The model under review builds one solid part; all positions refer to its coordinate system, in mm. Round coordinates to 2 decimals unless told otherwise and drop trailing zeros. Write each loop counter-clockwise with the first axis right and the second up, starting at its lowest first coordinate (ties: lowest second). Pieces come first, ordered by that corner, then holes. Notation, with made-up numbers: M 39.5,-13 L 61.5,-13 A28 cw 61.5,8 Z; hole C -8.75,7.25 d3. An arc over 180 degrees is marked long. Write item = value, one per line. Start each with the question number.
Item 1: Take a section at A-A, the plane x = 43.5. Give the boundary of the cut face in (y, z), plus the area to 3 significant figures.
Item 2: To check wall thickness, follow line 1 along X through (y, z) = (32, 78); line 2 along X through (y, z) = (31.45, 78); line 3 along X through (y, z) = (31.8, 93). State the ranges of each line that lie inside material, in increasing order.
Item 3: Take a section at C-C, the plane x = 68.5. Give the boundary of the cut face in (y, z).
Item 4: For pin 1 Ø2 at (x, z) = (43.5, 3.5) entering from -Y, flat-tipped, find the tip position at first contact; note if it passes through.
Item 5: Take a section at D-D, the plane y = 31.05. Give the boundary of the cut face in (x, z).
Item 6: Take a section at B-B, the plane z = 102.5. Give the boundary of the cut face in (x, y).
from build123d import *
from build123d.topology import SkipClean

# Parameters (mm, degrees)
SKETCH1_R                      = 40
SKETCH1_R_2                    = 38
BOSS_EXTRUDE1_DEPTH            = 200
SKETCH2_R                      = 40
BOSS_EXTRUDE2_DEPTH            = 2
BOSS_EXTRUDE3_DEPTH            = 107
BOSS_EXTRUDE4_DEPTH            = 2
SKETCH5_R                      = 1.75
CUT_EXTRUDE1_DEPTH             = 226.077764339
CUT_EXTRUDE2_REACH             = 218.296
SKETCH6_R                      = 4
CUT_EXTRUDE2_DIRECTION_2_REACH = 218.296
CIRPATTERN1_COUNT              = 2
CIRPATTERN1_ANGLE              = 90
BOSS_EXTRUDE5_REACH            = 241.742
BOSS_EXTRUDE5_END_RADIUS       = 40
SKETCH7_W                      = 14
SKETCH7_H                      = 2
CUT_EXTRUDE3_REACH             = 221.073
SKETCH8_R                      = 1.75
FILLET1_R                      = 3
CUT_EXTRUDE4_REACH             = 220.598
SKETCH9_R                      = 0.25
BOSS_EXTRUDE6_START            = 2
BOSS_EXTRUDE6_DEPTH            = 2
SKETCH11_R                     = 38
CUT_EXTRUDE5_DEPTH             = 219.146739623
CUT_EXTRUDE6_DEPTH             = 2


with BuildPart() as part:
    # Sketch1 → Boss-Extrude1 (new body)
    with BuildSketch(Plane.XY):
        Circle(SKETCH1_R)
        Circle(SKETCH1_R_2, mode=Mode.SUBTRACT)
    extrude(amount=BOSS_EXTRUDE1_DEPTH)

    # Sketch2 → Boss-Extrude2 (add)
    with BuildSketch(Plane.XY.offset(180)):
        Circle(SKETCH2_R)
    extrude(amount=BOSS_EXTRUDE2_DEPTH)

    # Sketch3 → Boss-Extrude3 (add)
    with BuildSketch(Plane(origin=(0, 0, 0), x_dir=(-1, 0, 0), z_dir=(0, 0, -1))):
        with BuildLine():
            Line((-21.071307506, -34), (-72, -34))
            Line((-72, -34), (-72, -30))
            Line((-72, -30), (-26.457513111, -30))
            ThreePointArc((-26.457513111, -30), (-23.848421275, -32.113125085), (-21.071307506, -34))
        make_face()
        with BuildLine():
            Line((-21.071307506, 34), (-72, 34))
            Line((-72, 34), (-72, 30))
            Line((-72, 30), (-26.457513111, 30))
            ThreePointArc((-26.457513111, 30), (-23.848421275, 32.113125085), (-21.071307506, 34))
        make_face()
    extrude(amount=-BOSS_EXTRUDE3_DEPTH)

    # Sketch4 → Boss-Extrude4 (add)
    with BuildSketch(Plane.XY.offset(107)):
        with BuildLine():
            Line((72, -34), (21.071307506, -34))
            ThreePointArc((21.071307506, -34), (40, 0), (21.071307506, 34))
            Line((21.071307506, 34), (72, 34))
            Line((72, 34), (72, -34))
        make_face()
    extrude(amount=BOSS_EXTRUDE4_DEPTH)

    # Sketch5 → Cut-Extrude1 (cut, through all)
    with BuildSketch(Plane(origin=(0, 34, 0), x_dir=(1, 0, 0), z_dir=(0, 1, 0))):
        with Locations(Location((43.5, -102.5, 0), (0, 0, 270))):
            Circle(SKETCH5_R)
        with Locations(Location((43.5, -3.5, 0), (0, 0, 270))):
            Circle(SKETCH5_R)
        with Locations(Location((68.5, -78, 0), (0, 0, 270))):
            Circle(SKETCH5_R)
    extrude(amount=-CUT_EXTRUDE1_DEPTH, mode=Mode.SUBTRACT)

    # Sketch6 → Cut-Extrude2 (cut, up to next)
    with BuildSketch(Plane(origin=(0, 0, 0), x_dir=(0, 0, 1), z_dir=(-0.7071067811865488, 0.7071067811865464, 0)), mode=Mode.PRIVATE) as cut_extrude2_sk1:
        with Locations(Location((187, 0, 0), (0, 0, 90))):
            Circle(SKETCH6_R)
    cut_extrude2_tool1 = extrude(cut_extrude2_sk1.sketch, amount=-CUT_EXTRUDE2_REACH, mode=Mode.PRIVATE) & part.part
    cut_extrude2 = cut_extrude2_tool1.solids().sort_by_distance((0, 0, 187))[0]
    add(cut_extrude2, mode=Mode.SUBTRACT)

    # Sketch6 → Cut-Extrude2 direction 2 (cut, up to next)
    with BuildSketch(Plane(origin=(0, 0, 0), x_dir=(0, 0, 1), z_dir=(-0.7071067811865488, 0.7071067811865464, 0)), mode=Mode.PRIVATE) as cut_extrude2_direction_2_sk1:
        with Locations(Location((187, 0, 0), (0, 0, 90))):
            Circle(SKETCH6_R)
    cut_extrude2_direction_2_tool1 = extrude(cut_extrude2_direction_2_sk1.sketch, amount=CUT_EXTRUDE2_DIRECTION_2_REACH, mode=Mode.PRIVATE) & part.part
    cut_extrude2_direction_2 = cut_extrude2_direction_2_tool1.solids().sort_by_distance((0, 0, 187))[0]
    add(cut_extrude2_direction_2, mode=Mode.SUBTRACT)

    # CirPattern1: Cut-Extrude2, Cut-Extrude2 direction 2 ×2 about axis
    cirpattern1_axis = Axis((0, 0, -5.35), (0, 0, 1))
    add([cut_extrude2.rotate(cirpattern1_axis, i * CIRPATTERN1_ANGLE / (CIRPATTERN1_COUNT - 1)) for i in range(1, CIRPATTERN1_COUNT)], mode=Mode.SUBTRACT)
    add([cut_extrude2_direction_2.rotate(cirpattern1_axis, i * CIRPATTERN1_ANGLE / (CIRPATTERN1_COUNT - 1)) for i in range(1, CIRPATTERN1_COUNT)], mode=Mode.SUBTRACT)

    # Boss-Extrude5: up to this cylinder (the profile starts outside it)
    boss_extrude5_end = Plane(origin=(0, 0, 7), z_dir=(0, 0, -1)) * Cylinder(BOSS_EXTRUDE5_END_RADIUS, 564.484, mode=Mode.PRIVATE)
    # Sketch7 → Boss-Extrude5 (add, up to the surface)
    with BuildSketch(Plane(origin=(-54, 0, 0), x_dir=(0, 0, -1), z_dir=(1, 0, 0)), mode=Mode.PRIVATE) as boss_extrude5_sk1:
        with Locations((-7, -12)):
            Rectangle(SKETCH7_W, SKETCH7_H)
    boss_extrude5_tool1 = extrude(boss_extrude5_sk1.sketch, amount=BOSS_EXTRUDE5_REACH, mode=Mode.PRIVATE) - boss_extrude5_end
    add(boss_extrude5_tool1.solids().sort_by_distance((-54, -12, 7))[0])
    # Sketch7 → Boss-Extrude5 (add, up to the surface)
    with BuildSketch(Plane(origin=(-54, 0, 0), x_dir=(0, 0, -1), z_dir=(1, 0, 0)), mode=Mode.PRIVATE) as boss_extrude5_sk2:
        with Locations((-7, 12)):
            Rectangle(SKETCH7_W, SKETCH7_H)
    boss_extrude5_tool2 = extrude(boss_extrude5_sk2.sketch, amount=BOSS_EXTRUDE5_REACH, mode=Mode.PRIVATE) - boss_extrude5_end
    add(boss_extrude5_tool2.solids().sort_by_distance((-54, 12, 7))[0])

    # Cut-Extrude3: up to this face of the body (flat: up to its plane)
    cut_extrude3_end = Plane(part.part.faces().sort_by_distance((-45.914280319, 13, 7))[0])
    # Sketch8 → Cut-Extrude3 (cut, up to the picked face)
    with BuildSketch(Plane.XZ.offset(13), mode=Mode.PRIVATE) as cut_extrude3_sk1:
        with Locations(Location((-49.770305539, 5.008755099, 0), (0, 0, 270))):
            Circle(SKETCH8_R)
    cut_extrude3_tool1 = split(extrude(cut_extrude3_sk1.sketch, amount=-CUT_EXTRUDE3_REACH, mode=Mode.PRIVATE), bisect_by=cut_extrude3_end, keep=Keep.BOTH, mode=Mode.PRIVATE)
    add(cut_extrude3_tool1.solids().sort_by(Axis((-49.770306, -13, 5.008755), (0, 1, 0)))[0], mode=Mode.SUBTRACT)

    # Fillet1
    fillet1_edges = [part.edges().sort_by_distance(p)[0] for p in [
        (-54, -12, 14),
        (-54, -12, 0),
        (-54, 12, 0),
        (-54, 12, 14),
    ]]
    fillet(fillet1_edges, radius=FILLET1_R)

    # Sketch9 → Cut-Extrude4 (cut, up to next)
    with BuildSketch(Plane.XZ.offset(-11), mode=Mode.PRIVATE) as cut_extrude4_sk1:
        with Locations(Location((-43.770305539, 7.008755099, 0), (0, 0, 270))):
            Circle(SKETCH9_R)
    cut_extrude4_tool1 = extrude(cut_extrude4_sk1.sketch, amount=-CUT_EXTRUDE4_REACH, mode=Mode.PRIVATE) & part.part
    add(cut_extrude4_tool1.solids().sort_by_distance((-43.770306, 11, 7.008755))[0], mode=Mode.SUBTRACT)

    # Sketch10 → Boss-Extrude6 (add)
    with SkipClean():  # the faces are left unmerged after this step: merging them gives an invalid solid
        with BuildSketch(Plane(origin=(0, 0, 0), x_dir=(-1, 0, 0), z_dir=(0, 0, -1)).offset(BOSS_EXTRUDE6_START)):
            with BuildLine():
                ThreePointArc((10, -36.66060556), (0, -38), (-10, -36.66060556))
                Line((-10, -36.66060556), (-10, -38.729833462))
                ThreePointArc((-10, -38.729833462), (0, -40), (10, -38.729833462))
                Line((10, -38.729833462), (10, -36.66060556))
            make_face()
            with BuildLine():
                ThreePointArc((10, 38.729833462), (0, 40), (-10, 38.729833462))
                Line((-10, 38.729833462), (-10, 36.66060556))
                ThreePointArc((-10, 36.66060556), (0, 38), (10, 36.66060556))
                Line((10, 36.66060556), (10, 38.729833462))
            make_face()
        extrude(amount=-BOSS_EXTRUDE6_DEPTH)

    # Sketch11 → Cut-Extrude5 (cut, through all)
    # profile 1 of 4: a face of its own
    with BuildSketch(Plane.XY.offset(200)):
        with BuildLine():
            ThreePointArc((-1.947772516, -39.952549133), (-40, 0), (-1.947772516, 39.952549133))
            ThreePointArc((-1.947772516, 39.952549133), (-79.070653643, 0), (-1.947772516, -39.952549133))
        make_face()
    # profile 2 of 4: a face of its own
    with BuildSketch(Plane.XY.offset(200)):
        with BuildLine():
            ThreePointArc((40, 0), (36.457513111, 16.457513111), (26.457513111, 30))
            ThreePointArc((26.457513111, 30), (23.848421275, 32.113125085), (21.071307506, 34))
            ThreePointArc((21.071307506, 34), (10.014270214, 38.726146104), (-1.947772516, 39.952549133))
            ThreePointArc((-1.947772516, 39.952549133), (-40, 0), (-1.947772516, -39.952549133))
            ThreePointArc((-1.947772516, -39.952549133), (10.014270214, -38.726146104), (21.071307506, -34))
            ThreePointArc((21.071307506, -34), (34.94890771, -19.456974325), (40, 0))
        make_face()
        Circle(SKETCH11_R, mode=Mode.SUBTRACT)
    # profile 3 of 4: a face of its own
    with BuildSketch(Plane.XY.offset(200)):
        with BuildLine():
            Line((72, -34), (72, 30))
            Line((72, 30), (26.457513111, 30))
            ThreePointArc((26.457513111, 30), (36.457513111, 16.457513111), (40, 0))
            ThreePointArc((40, 0), (34.94890771, -19.456974325), (21.071307506, -34))
            Line((21.071307506, -34), (72, -34))
        make_face()
    # profile 4 of 4: a face of its own
    with BuildSketch(Plane.XY.offset(200)):
        Circle(SKETCH11_R)
    extrude(amount=-CUT_EXTRUDE5_DEPTH, mode=Mode.SUBTRACT)

    # Sketch12 → Cut-Extrude6 (cut)
    with BuildSketch(Plane.XY.offset(109)):
        with BuildLine():
            Line((26.457513111, 30), (72, 30))
            Line((72, 30), (72, 34))
            Line((72, 34), (21.071307506, 34))
            ThreePointArc((21.071307506, 34), (23.848421275, 32.113125085), (26.457513111, 30))
        make_face()
    extrude(amount=-CUT_EXTRUDE6_DEPTH, mode=Mode.SUBTRACT)


solid = part.part
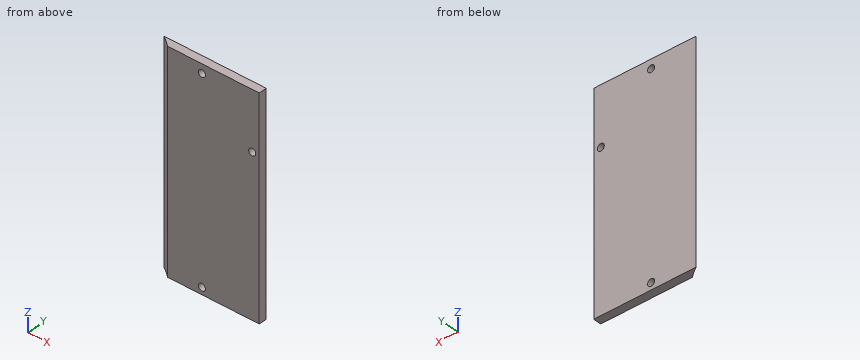
Response values:
q1.outline = M 30,0 L 34,0 L 34,1.75 L 30,1.75 Z; M 30,5.25 L 34,5.25 L 34,100.75 L 30,100.75 Z; M 30,104.25 L 34,104.25 L 34,107 L 30,107 Z
q1.area = 400 mm2
q2.line_1 = 24 to 66.75, 70.25 to 72
q2.line_2 = 24.72 to 66.75, 70.25 to 72
q2.line_3 = 24.26 to 72
q3.outline = M 30,0 L 34,0 L 34,76.25 L 30,76.25 Z; M 30,79.75 L 34,79.75 L 34,107 L 30,107 Z
q4.pin_1 = through
q5.outline = M 25.22,0 L 72,0 L 72,107 L 25.22,107 Z; hole C 43.5,3.5 d3.5; hole C 43.5,102.5 d3.5; hole C 68.5,78 d3.5
q6.outline = M 21.07,34 A40 cw 26.46,30 L 41.75,30 L 41.75,34 Z; M 45.25,30 L 72,30 L 72,34 L 45.25,34 Z
